Work out the finished part from the listing and answer in its coordinate system (mm). A direction names the side the tool comes from. Coordinates: 2 decimals unless noted, no trailing zeros. Loops run counter-clockwise (first coordinate to the right, second up) from the corner with the lowest first, then second, coordinate; pieces in that order, holes last. Notation, with made-up numbers: (78, -32) -> (104, -32) arc R13 ccw to (104, -26) -> close; hole circle Ø7 at (57, -26). An arc over 180 degrees is marked (long way). Use a Markdown table: item, result.
Autodesk Inventor part; units mm, degrees
ref_plane "YZ Plane" through (0, 0, 0) normal (1, 0, 0) x (0, 1, 0)
ref_plane "XZ Plane" through (0, 0, 0) normal (0, 1, 0) x (-1, 0, 0)
ref_plane "XY Plane" through (0, 0, 0) normal (0, 0, 1) x (1, 0, 0)
sketch "Sketch1" plane through (0, 0, 0) normal (0, 1, 0) x (-1, 0, 0)
  line L0 (0, 0) -> (-100, 0) construction
  line L1 (-100, 0) -> (-100, 100)
  line L2 (-100, 100) -> (0, 100)
  line L3 (0, 100) -> (0, 0)
  circle A0 centre (-4.25, 92) radius 0.575
  circle A1 centre (-4.25, 74) radius 0.575
  line L4 (-50, 100) -> (-50, 0) construction
  line L5 (-7.212, 23.8876) -> (-7.212, 67.0676) construction
  line L6 (-7.212, 67.0676) -> (-43.788, 67.0676) construction
  line L7 (-7.212, 23.8876) -> (-43.788, 23.8876) construction
  circle A2 centre (-7.212, 67.0676) radius 1.5
  circle A3 centre (-43.788, 67.0676) radius 1.5
  circle A4 centre (-7.212, 23.8876) radius 1.5
  circle A5 centre (-43.788, 23.8876) radius 1.5
  line L8 (-43.788, 9.0676) -> (-92.788, 9.0676) construction
  line L9 (-92.788, 9.0676) -> (-92.788, 67.0676) construction
  line L10 (-92.788, 67.0676) -> (-43.788, 67.0676) construction
  line L11 (-43.788, 67.0676) -> (-43.788, 9.0676) construction
  circle A6 centre (-43.788, 9.0676) radius 1.375
  circle A7 centre (-92.788, 9.0676) radius 1.375
  circle A8 centre (-92.788, 67.0676) radius 1.375
  circle A9 centre (-43.788, 67.0676) radius 1.375
  line L12 (-7.212, 45.4776) -> (0, 45.4776) construction
  line L13 (-92.788, 38.0676) -> (-100, 38.0676) construction
  circle A10 centre (-43.269, 0) radius 1.143
  line L14 (0, 0) -> (-100, 0) construction
  circle A11 centre (-95.75, 74) radius 0.575
  circle A12 centre (-56.731, 0) radius 1.143
  circle A13 centre (-95.75, 92) radius 0.575
  line L15 (-39, 7) -> (-61, 7)
  line L16 (-61, 7) -> (-61, -7)
  line L17 (-61, -7) -> (-39, -7)
  line L18 (-39, -7) -> (-39, 7)
  line L19 (-39, 7) -> (-61, -7) construction
  line L20 (-61, 7) -> (-39, -7) construction
  line L21 (-50, 0) -> (-50, -25) construction
  line L22 (-50, -25) -> (-20.9775, -25)
  line L23 (-20.9775, -25) -> (0, 0)
  line L24 (-7.8324, 0) -> (-23.7753, -19)
  line L25 (-23.7753, -19) -> (-50, -19)
  line L26 (-39, 7) -> (-16.1201, 7)
  line L27 (-16.1201, 7) -> (-7.8324, 0)
  line L28 (-50, -25) -> (-79.0225, -25)
  line L29 (-79.0225, -25) -> (-100, 0)
  line L30 (-92.1676, 0) -> (-76.2247, -19)
  line L31 (-76.2247, -19) -> (-50, -19)
  line L32 (-61, 7) -> (-83.8799, 7)
  line L33 (-83.8799, 7) -> (-92.1676, 0)
  line L34 (-30, 100) -> (-70, 100)
  point P0 (-50, 80)
  dimension "d0" = 100
  dimension "d1" = 100
  dimension "d2" = 8
  dimension "d3" = 4.25
  dimension "d4" = 1.15
  dimension "d5" = 18
  dimension "d6" = 43.18
  dimension "d7" = 36.576
  dimension "d8" = 3
  dimension "d9" = 49
  dimension "d10" = 58
  dimension "d15" = 2.75
  dimension "d16" = 13.462
  dimension "d17" = 2.286
  dimension "d33" = 22
  dimension "d34" = 25
  dimension "d36" = 130
  dimension "d37" = 6
  dimension "d38" = 6
  dimension "d39" = 14
extrude "Extrusion1" add sketch "Sketch1" along normal blind 3 contours L1 L2 L3 L23 L22 L28 L29 | L18 L17 L16 L15
fillet "Fillet1" radius 6 10 edges at (61, 1.5, 7) (39, 1.5, 7) (39, 1.5, -7) (61, 1.5, -7) (7.8324, 1.5, 0) (92.1676, 1.5, 0) (83.8799, 1.5, 7) (16.1201, 1.5, 7) (23.7753, 1.5, -19) (76.2247, 1.5, -19)
fillet "Fillet1" radius 8 6 edges at (20.9775, 1.5, -25) (0, 1.5, 0) (79.0225, 1.5, -25) (100, 1.5, 0) (100, 1.5, 100) (0, 1.5, 100)
properties part number "ROBOT CHASSIS PLATE"
Q1. Consider line 1 (X direction, y = 1.4, z = 92) (3 decimals); line 2 (Z direction, x = 57.5, y = 1.9); line 3 (Z direction, x = 47.5, y = 2.6). Determine where each line is inside the solid, lowest interval first. Write a range as [from, to].
Solved:
| item | result |
|---|---|
| line 1 | [0, 3.675], [4.825, 95.175], [96.325, 100] |
| line 2 | [-25, -19], [-6.45, -0.85], [0.85, 100] |
| line 3 | [-25, -19], [-7, 100] |
Q2. Given pin 1 Ø1.5 at (x, y) = (23.5, 2) entering from -Z, flat-ended and moving along its own axis, determine where the tip first touches the part or whether it passes through.
Solved:
| item | result |
|---|---|
| pin 1 | z = -24.99 |
Q3. For faces 1 (the flat face through (51, 0, 52)), 2 (the cylindrical face through (59.289, 1.521, -5.196)), determine the directions among +Z, -Z, +X, -X, +Y, -Y from which every point of the face is accessible in a straight line to the end or side of a thin tool.
Solved:
| item | result |
|---|---|
| face 1 | +Z, -Z, +X, -X, -Y |
| face 2 | +Y, -Y |
Q4. Section A-A on x = 65 is taken. Determine the outline of the cut face in (y, z).
Solved:
| item | result |
|---|---|
| outline | (0, -25) -> (3, -25) -> (3, -19) -> (0, -19) -> close; (0, 6.66) -> (3, 6.66) -> (3, 100) -> (0, 100) -> close |
Q5. Section B-B on y = 0.7 is taken. State how many separate pieces and enclosed holes the cut face has, and give its area (3 significant figures).
Solved:
| item | result |
|---|---|
| separate pieces | 1 |
| enclosed holes | 14 |
| area | 10,400 mm² |
Q6. Determine the mould class of faces 3 (the flat face through (51, 1, 100)), 4 (the cylindrical face through (6.41, 1.48, 65.8)), 5 (the flat face through (50, 1, -25)), 6 (the cylindrical face through (45.287, 1.479, 23.822)) for opening direction Z: pulls with the +Z half, pulls with the -Z half, needs draft (parallel to the pull), parting line crosses it, or undercut.
Solved:
| item | result |
|---|---|
| face 3 | pulls with the +Z half |
| face 4 | undercut |
| face 5 | pulls with the -Z half |
| face 6 | undercut |
